Can you work these out from the drawing? Everything is in mm from the part's minimum corner. Give positions to 0.01 mm unless a question says otherwise; leave off trailing zeros. Loops run counter-clockwise (first coordinate to the right, second up) from the corner with the lowest first, then second, coordinate; pieces in that order, holes last.
Q1. Will these pins go through, and if not, where does the flat tip stop? P1, Ø1, axis at y = 2, z = 3, coming from the +X side (1 decimal); P2, Ø1, axis at y = 6.5, z = 12, coming from the -X side; P3, Ø2, axis at x = 2.5, z = 7.5, coming from the -Y side.
Q2. I need wall thicknesses on line 1 (Y direction, x = 3, z = 10.5) (1 decimal); line 2 (Y direction, x = 5.25, z = 18.5) (1 decimal); line 3 (X direction, y = 3.5, z = 15) (1 decimal). Which ranges of each line are inside material? Lowest first, please.
Q3. If we section it at B-B (z = 1.5): Please give me the cut outline in (x, y).
Q4. We'd pull the mould along Y, two halves only. Please class the marked faces 1, 2 and 3: +Y half, -Y half, draft (parallel to the pull), parting line (faces both ways), or undercut.
Q5. If we section it at A-A (z = 13.25): Please give me the cut outline in (x, y).
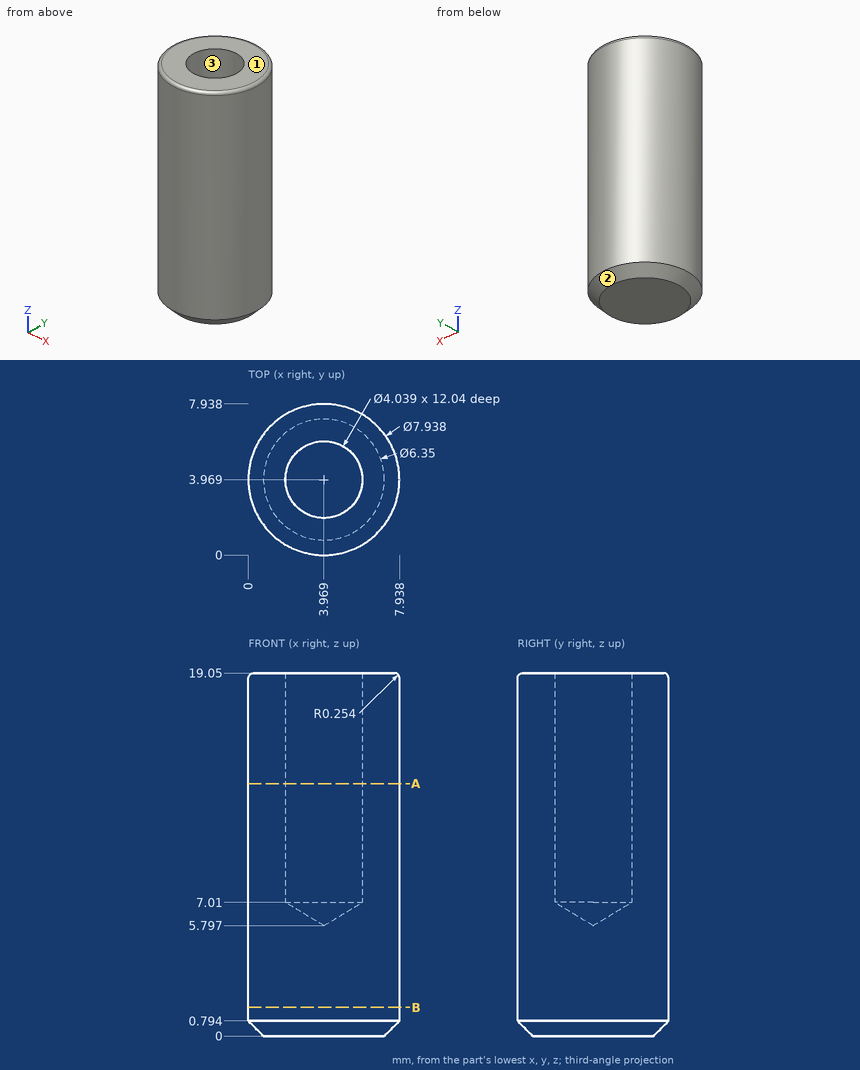
Check sheet entries:
1. P1: stops at x = 7.7
1. P2: stops at x = 0.56
1. P3: stops at y = 0.03
2. line 1: y = 0.1 to 2.2, 5.7 to 7.8
2. line 2: y = 0.2 to 2.4, 5.5 to 7.7
2. line 3: x = 0 to 2, 5.9 to 7.9
3. outline: circle Ø7.94 at (3.97, 3.97)
4. face 1: draft
4. face 2: parting line
4. face 3: undercut
5. outline: circle Ø7.94 at (3.97, 3.97); hole circle Ø4.04 at (3.97, 3.97)
